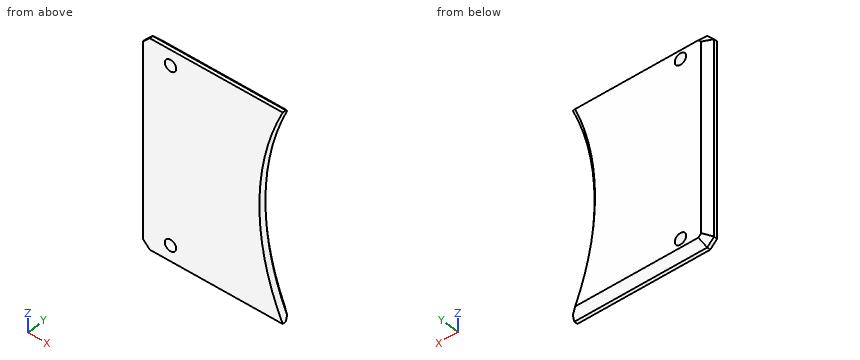
from build123d import *

# Parameters (mm, degrees)
ESQUISSE1_R        = 1.65
BOSS_EXTRU_1_DEPTH = 3
CHANFREIN1_SIZE    = 2
CHANFREIN3_SIZE    = 2
CHANFREIN4_SIZE    = 1


with BuildPart() as part:
    # Esquisse1 → Boss.-Extru.1 (new body)
    with BuildSketch(Plane(origin=(0, 0, 0), x_dir=(1, 0, 0), z_dir=(0, 1, 0))):
        with BuildLine():
            Line((-20.25, -30), (20.25, -30))
            ThreePointArc((20.25, -30), (13.495553203, 0), (20.25, 30))
            Line((20.25, 30), (-20.25, 30))
            Line((-20.25, 30), (-20.25, -30))
        make_face()
        with Locations(Location((-12.25, -25.5, 0), (0, 0, 270))):
            Circle(ESQUISSE1_R, mode=Mode.SUBTRACT)
        with Locations(Location((-12.25, 25.5, 0), (0, 0, 270))):
            Circle(ESQUISSE1_R, mode=Mode.SUBTRACT)
    extrude(amount=-BOSS_EXTRU_1_DEPTH)

    # Chanfrein1
    chanfrein1_edges = [part.edges().sort_by_distance(p)[0] for p in [
        (-20.25, -1.5, 30),
        (-20.25, -1.5, -30),
    ]]
    chamfer(chanfrein1_edges, length=CHANFREIN1_SIZE)

    # Chanfrein3
    chanfrein3_edges = [part.edges().sort_by_distance(p)[0] for p in [
        (-20.25, 0, 0),
        (1, 0, 30),
        (-19.25, 0, -29),
        (-19.25, 0, 29),
        (1, 0, -30),
    ]]
    chamfer(chanfrein3_edges, length=CHANFREIN3_SIZE)

    # Chanfrein4
    chanfrein4_edges = [part.edges().sort_by_distance(p)[0] for p in [
        (13.495553203, 0, 0),
    ]]
    chamfer(chanfrein4_edges, length=CHANFREIN4_SIZE)


solid = part.part
Read the model definition and answer for the solid it produces. Units are mm, in the model's axes. Round coordinates to 2 decimals unless told otherwise and drop trailing zeros. Write each loop counter-clockwise with the first axis right and the second up, starting at its lowest first coordinate (ties: lowest second). Pieces come first, ordered by that corner, then holes.
Q1. Find section A-A on x = -12.25. Determine the outline of the cut face in (y, z).
Values:
outline: (-3, -30) - (-2, -30) - (0, -28) - (0, -27.15) - (-3, -27.15) - close; (-3, -23.85) - (0, -23.85) - (0, 23.85) - (-3, 23.85) - close; (-3, 27.15) - (0, 27.15) - (0, 28) - (-2, 30) - (-3, 30) - close
Q2. Find section C-C on x = 0. Determine the outline of the cut face in (y, z).
Values:
outline: (-3, -30) - (-2, -30) - (0, -28) - (0, 28) - (-2, 30) - (-3, 30) - close
Q3. Flat-ended cylindrical pins translate along their axes: P1, Ø4, axis at x = -12.25, z = 25.5, coming from the +Y side; P2, Ø1.5, axis at y = -1, z = -17, coming from the -X side. Find the tip coordinate at first contact, or state that the pin passes through.
Values:
P1: stops at y = 0
P2: stops at x = -20
Q4. Straight lines are drawn through the part: line 1 (X direction, y = -0.65, z = 25.5); line 2 (X direction, y = -1.4, z = 25.5); line 3 (X direction, y = -0.75, z = 3). For each, find the intervals that lie inside material, in ascending order.
Values:
line 1: x = -18.9 to -13.9, -10.6 to 17.93
line 2: x = -19.65 to -13.9, -10.6 to 18.31
line 3: x = -19 to 13.31
Q5. Find section B-B on y = -0.5. Determine the outline of the cut face in (x, z), and give its area (3 significant figures).
Values:
outline: (-18.75, -27.38) - (-17.63, -28.5) - (19.01, -28.5) arc R70.5 cw to (19.01, 28.5) - (-17.63, 28.5) - (-18.75, 27.38) - close; hole circle Ø3.3 at (-12.25, -25.5); hole circle Ø3.3 at (-12.25, 25.5)
area: 1,900 mm2
